Work out the finished part from the listing and answer in its coordinate system (mm). Round coordinates to 2 decimals unless told otherwise and drop trailing zeros. Order: outer loops, then holes, each group sorted by start corner. A loop starts at its lowest first (then second) coordinate and runs counter-clockwise, first axis right, second up. Notation, with made-up numbers: (-8.75, -30) - (-0.75, -30) arc R9 ccw to (-0.75, -25) - close; hole circle Ø2 at (59.25, -29). An arc over 180 degrees is marked (long way). Use one line per item in the form item = value. Start each with the question number.
Q1. The part is cut by section A-A on x = 191. Determine the outline of the cut face in (y, z).
Q2. Given P1, Ø1.2, axis at x = 251.5, z = -32.5, coming from the -Y side; P2, Ø2, axis at y = 80.5, z = -31.5, coming from the -X side; P3, Ø1, axis at y = 34.5, z = -33, coming from the +X side, each flat-ended and moving along its own axis, determine where each tip first touches the part or whether it passes through.
Q3. Find the intervals of material crossed by line 1 (Y direction, x = 242.5, z = -31); line 2 (Y direction, x = 151, z = -31.75); line 3 (Z direction, x = 151, y = 4.7), in increasing order. Write a range as [from, to].
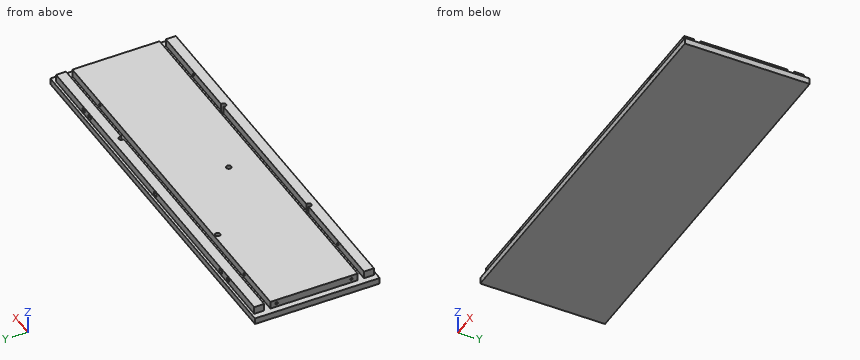
from build123d import *

# Parameters (mm, degrees)
SKETCH002_W     = 312
SKETCH002_H     = 100
PAD002_DEPTH    = 11
SKETCH003_W     = 312
SKETCH003_H     = 2
POCKET_DEPTH    = 6
SKETCH004_W     = 5
SKETCH004_H     = 96
POCKET001_DEPTH = 6
SKETCH008_W     = 302
SKETCH008_H     = 5
POCKET003_DEPTH = 6
SKETCH018_R     = 2
POCKET011_DEPTH = 5
SKETCH019_R     = 2
POCKET012_DEPTH = 5
SKETCH020_R     = 1
POCKET013_DEPTH = 15
SKETCH021_R     = 1
POCKET014_DEPTH = 15
SKETCH022_R     = 1
POCKET015_DEPTH = 20
SKETCH023_R     = 1
POCKET016_DEPTH = 20
CHAMFER001_SIZE = 0.8
SKETCH058_R     = 2
POCKET028_DEPTH = 8


with BuildPart() as part:
    # Sketch002 → Pad002 (new body)
    with BuildSketch(Plane.XY):
        with Locations((156, 50)):
            Rectangle(SKETCH002_W, SKETCH002_H)
    extrude(amount=PAD002_DEPTH)

    # Sketch003 (on Face6 of Pad002) → Pocket (cut)
    with BuildSketch(Plane.XY.offset(11)):
        with Locations((156, 1)):
            Rectangle(SKETCH003_W, SKETCH003_H)
        with Locations((156, 99)):
            Rectangle(SKETCH003_W, SKETCH003_H)
    extrude(amount=-POCKET_DEPTH, mode=Mode.SUBTRACT)

    # Sketch004 (on Face9 of Pocket) → Pocket001 (cut)
    with BuildSketch(Plane.XY.offset(11)):
        with Locations((2.5, 50)):
            Rectangle(SKETCH004_W, SKETCH004_H)
        with Locations((309.5, 50)):
            Rectangle(SKETCH004_W, SKETCH004_H)
    extrude(amount=-POCKET001_DEPTH, mode=Mode.SUBTRACT)

    # Sketch008 (on Face13 of Pocket001) → Pocket003 (cut)
    with BuildSketch(Plane.XY.offset(11)):
        with Locations((156, 87.5)):
            Rectangle(SKETCH008_W, SKETCH008_H)
        with Locations((156, 12.5)):
            Rectangle(SKETCH008_W, SKETCH008_H)
    extrude(amount=-POCKET003_DEPTH, mode=Mode.SUBTRACT)

    # Sketch018 (on Face9 of Pocket003) → Pocket011 (cut)
    with BuildSketch(Plane.XZ.offset(-2)):
        with Locations((56, 8)):
            Circle(SKETCH018_R)
        with Locations((156, 8)):
            Circle(SKETCH018_R)
        with Locations((256, 8)):
            Circle(SKETCH018_R)
    extrude(amount=-POCKET011_DEPTH, mode=Mode.SUBTRACT)

    # Sketch019 (on Face11 of Pocket011) → Pocket012 (cut)
    with BuildSketch(Plane(origin=(0, 98, 0), x_dir=(-1, 0, 0), z_dir=(0, 1, 0))):
        with Locations((-56, 8)):
            Circle(SKETCH019_R)
        with Locations((-156, 8)):
            Circle(SKETCH019_R)
        with Locations((-256, 8)):
            Circle(SKETCH019_R)
    extrude(amount=-POCKET012_DEPTH, mode=Mode.SUBTRACT)

    # Sketch020 (on Face22 of Pocket012) → Pocket013 (cut)
    with BuildSketch(Plane(origin=(5, 0, 0), x_dir=(0, -1, 0), z_dir=(-1, 0, 0))):
        with Locations((-20, 8)):
            Circle(SKETCH020_R)
        with Locations((-80, 8)):
            Circle(SKETCH020_R)
    extrude(amount=-POCKET013_DEPTH, mode=Mode.SUBTRACT)

    # Sketch021 (on Face14 of Pocket013) → Pocket014 (cut)
    with BuildSketch(Plane.YZ.offset(307)):
        with Locations((80, 8)):
            Circle(SKETCH021_R)
        with Locations((20, 8)):
            Circle(SKETCH021_R)
    extrude(amount=-POCKET014_DEPTH, mode=Mode.SUBTRACT)

    # Sketch022 (on Face9 of Pocket014) → Pocket015 (cut)
    with BuildSketch(Plane.XZ.offset(-2)):
        with Locations((45, 8)):
            Circle(SKETCH022_R)
        with Locations((265, 8)):
            Circle(SKETCH022_R)
    extrude(amount=-POCKET015_DEPTH, mode=Mode.SUBTRACT)

    # Sketch023 (on Face11 of Pocket015) → Pocket016 (cut)
    with BuildSketch(Plane(origin=(0, 98, 0), x_dir=(-1, 0, 0), z_dir=(0, 1, 0))):
        with Locations((-45, 8)):
            Circle(SKETCH023_R)
        with Locations((-265, 8)):
            Circle(SKETCH023_R)
    extrude(amount=-POCKET016_DEPTH, mode=Mode.SUBTRACT)

    # Chamfer001
    chamfer001_edges = [part.edges().sort_by_distance(p)[0] for p in [
        (46, 98, 8),
        (266, 98, 8),
        (264, 2, 8),
        (44, 2, 8),
    ]]
    chamfer(chamfer001_edges, length=CHAMFER001_SIZE)

    # Sketch058 (on Face3 of Chamfer001) → Pocket028 (cut)
    with BuildSketch(Plane.XY.offset(11)):
        with Locations((91, 9)):
            Circle(SKETCH058_R)
        with Locations((221, 9)):
            Circle(SKETCH058_R)
        with Locations((156, 39)):
            Circle(SKETCH058_R)
        with Locations((91, 82)):
            Circle(SKETCH058_R)
        with Locations((221, 91)):
            Circle(SKETCH058_R)
    extrude(amount=-POCKET028_DEPTH, mode=Mode.SUBTRACT)


with BuildPart() as part_1:
    # Body001 placement: moved
    add(part.part.moved(Location((-5, 0, -40))))


solid = part_1.part
Found:
q1.outline = (0, -40) - (100, -40) - (100, -35) - (98, -35) - (98, -29) - (90, -29) - (90, -35) - (85, -35) - (85, -29) - (15, -29) - (15, -35) - (10, -35) - (10, -29) - (2, -29) - (2, -35) - (0, -35) - close
q2.P1 = 7
q2.P2 = 0
q2.P3 = 302
q3.line_1 = [2, 10], [15, 85], [90, 98]
q3.line_2 = [7, 10], [15, 37], [41, 85], [90, 93]
q3.line_3 = [-40, -34], [-30, -29]
